Geometry check sheet. Reference: the model listing, model coordinates, mm. A direction names the side the tool comes from. Round coordinates to 2 decimals unless told otherwise and drop trailing zeros. Loops run counter-clockwise (first coordinate to the right, second up) from the corner with the lowest first, then second, coordinate; pieces in that order, holes last. Notation, with made-up numbers: (11, 63.25) -> (36, 63.25) arc R21 cw to (36, 101.25) -> close; hole circle Ø4 at (78.5, 56). An arc over 180 degrees is marked (long way). Use one line per item in the form item = value.
from build123d import *

# Parameters (mm, degrees)
SURFACE_EXTRUDE1_1_BACK  = 150
SURFACE_EXTRUDE1_1_DEPTH = 150
THICKEN1_T1              = 1
THICKEN1_T2              = 1
F_4_0MM_DOWEL_HOLE1_D    = 4


with BuildPart() as body_1:
    # Surface-Extrude1: a surface, the sketch's curves swept straight by 150 mm
    with BuildLine(Plane(origin=(0, 0, 0), x_dir=(0, 0, -1), z_dir=(1, 0, 0)).offset(-SURFACE_EXTRUDE1_1_BACK), mode=Mode.PRIVATE) as surface_extrude1_1_path:
        Line((0, 0), (-10, 0))
        Line((-10, 0), (-10, -12))
        Line((-10, -12), (0, -12))
    surface_extrude1_1 = Shell.extrude(surface_extrude1_1_path.wire(), (1 * SURFACE_EXTRUDE1_1_DEPTH, 0 * SURFACE_EXTRUDE1_1_DEPTH, 0 * SURFACE_EXTRUDE1_1_DEPTH))
    add(Solid.thicken(surface_extrude1_1, THICKEN1_T1))
    add(Solid.thicken(surface_extrude1_1, -THICKEN1_T2))

    # Ø4.0mm Dowel Hole1 (through all)
    with Locations(Plane(origin=(0, 1, 0), x_dir=(1, 0, 0), z_dir=(0, 1, 0))):
        with Locations((-125, -5.5), (-75, -5.5), (-25, -5.5)):
            Hole(F_4_0MM_DOWEL_HOLE1_D / 2)


solid = body_1.part
1. Mould release check, pull along Z, two halves, no side actions. Record for faces 1 (the flat face through (-76, 1, 8)), 2 (the flat face through (-76, -6, 11)), 3 (the cylindrical face through (-123.002, -0.014, 5.412)), 4 (the flat face through (-76, -6, 9)): released by +Z, released by -Z, zero draft, split by the parting line, or undercut.
Return value:
face_1 = zero draft
face_2 = released by +Z
face_3 = undercut
face_4 = released by -Z
2. Material ranges on line 1 along Z through (x, y) = (-25, -12.25); line 2 along Y through (x, z) = (-84.5, 3); line 3 along X through (y, z) = (-11.75, 7.25), recorded low to high.
Return value:
line_1 = 0 to 3.5, 7.5 to 11
line_2 = -13 to -11, -1 to 1
line_3 = -150 to -125.97, -124.03 to -75.97, -74.03 to -25.97, -24.03 to 0
3. Gauge pin test, flat ends, axial feed: pin 1 (3.5 mm diameter, centred on x = -75, z = 5.5, fed in from -Y); pin 2 (1 mm diameter, centred on x = -104, y = -7, fed in from -Z). Record the tip position at first contact, or that the pin passes through.
Return value:
pin_1 = through
pin_2 = 9
4. Section check A-A (z = 1.5). Record the boundary of the cut face in (x, y), then the cut area to 3 significant figures.
Return value:
outline = (-150, -13) -> (0, -13) -> (0, -11) -> (-150, -11) -> close; (-150, -1) -> (0, -1) -> (0, 1) -> (-150, 1) -> close
area = 600 mm2
5. Section check B-B (x = -25). Record the boundary of the cut face in (y, z).
Return value:
outline = (-13, 0) -> (-11, 0) -> (-11, 3.5) -> (-13, 3.5) -> close; (-13, 7.5) -> (-11, 7.5) -> (-11, 9) -> (-1, 9) -> (-1, 7.5) -> (1, 7.5) -> (1, 11) -> (-13, 11) -> close; (-1, 0) -> (1, 0) -> (1, 3.5) -> (-1, 3.5) -> close
6. Tool access check on faces 5 (the flat face through (-76, -1, 3)), 6 (the cylindrical face through (-76.908, -12.014, 4.899)). Record the directions out of +Z, -Z, +X, -X, +Y, -Y that give a thin tool (end or side, any length) a straight path to the whole face; none if there is none.
Return value:
face_5 = -Z, +X, -X
face_6 = +Y, -Y
7. Section check D-D (y = -5.5). Record the boundary of the cut face in (x, z).
Return value:
outline = (-150, 9) -> (0, 9) -> (0, 11) -> (-150, 11) -> close
8. Section check C-C (x = -80.5). Record the boundary of the cut face in (y, z).
Return value:
outline = (-13, 0) -> (-11, 0) -> (-11, 9) -> (-1, 9) -> (-1, 0) -> (1, 0) -> (1, 11) -> (-13, 11) -> close
